Source: CAD feature listing. Evaluate the final solid. Frame: model axes, mm. A direction names the side the tool comes from. Give positions to 0.01 mm unless a question says otherwise; leave off trailing zeros. Write each loop counter-clockwise with the first axis right and the second up, starting at its lowest first coordinate (ties: lowest second). Pieces come first, ordered by that corner, then holes. Notation, with made-up numbers: (38.25, 26.5) -> (78.25, 26.5) arc R33 ccw to (78.25, 63.5) -> close; hole circle Ø10 at (70.5, 32). An arc over 180 degrees is marked (long way). Write item = value, one per line.
from build123d import *

# Parameters (mm, degrees)
SKETCH_W        = 18.5
SKETCH_H        = 18.5
PAD_DEPTH       = 5.5
SKETCH001_W     = 15.5
SKETCH001_H     = 15.5
POCKET_DEPTH    = 4
SKETCH002_R     = 2.7059
PAD001_DEPTH    = 4
POCKET001_DEPTH = 4
FILLET001_R     = 1.5
FILLET_R        = 2
PAD002_DEPTH    = 1.35295
FILLET002_R     = 1


with BuildPart() as part:
    # Sketch → Pad (new body)
    with BuildSketch(Plane.XY):
        Rectangle(SKETCH_W, SKETCH_H)
    extrude(amount=PAD_DEPTH)

    # Sketch001 → Pocket (cut)
    with BuildSketch(Plane(origin=(0, 0, 0), x_dir=(1, 0, 0), z_dir=(0, 0, -1))):
        Rectangle(SKETCH001_W, SKETCH001_H)
    extrude(amount=-POCKET_DEPTH, mode=Mode.SUBTRACT)

    # Sketch002 (on Face11 of Pocket) → Pad001 (join)
    with BuildSketch(Plane(origin=(0, 0, 4), x_dir=(1, 0, 0), z_dir=(0, 0, -1))):
        Circle(SKETCH002_R)
    extrude(amount=PAD001_DEPTH)

    # Sketch003 (on Face13 of Pad001) → Pocket001 (cut)
    with BuildSketch(Plane(origin=(0, 0, 0), x_dir=(1, 0, 0), z_dir=(0, 0, -1))):
        Polygon((-0.6219, 2.0443), (0.6219, 2.0443), (0.6219, 0.6219), (2.0443, 0.6219), (2.0443, -0.6219), (0.6219, -0.6219), (0.6219, -2.0443), (-0.6219, -2.0443), (-0.6219, -0.6219), (-2.0443, -0.6219), (-2.0443, 0.6219), (-0.6219, 0.6219), align=None)
    extrude(amount=-POCKET001_DEPTH, mode=Mode.SUBTRACT)

    # Fillet001
    fillet001_edges = [part.edges().sort_by_distance(p)[0] for p in [
        (-7.75, -7.75, 2),
        (7.75, -7.75, 2),
        (7.75, 7.75, 2),
        (-7.75, 7.75, 2),
    ]]
    fillet(fillet001_edges, radius=FILLET001_R)

    # Fillet
    fillet_edges = [part.edges().sort_by_distance(p)[0] for p in [
        (9.25, -9.25, 2.75),
        (-9.25, -9.25, 2.75),
        (-9.25, 9.25, 2.75),
        (9.25, 9.25, 2.75),
    ]]
    fillet(fillet_edges, radius=FILLET_R)

    # Sketch004 (on Face19 of Fillet) → Pad002 (join)
    with BuildSketch(Plane(origin=(0, 0, 4), x_dir=(1, 0, 0), z_dir=(0, 0, -1))):
        Polygon((-0.676475, 7.75), (0.676475, 7.75), (0.676475, 0.676475), (7.75, 0.676475), (7.75, -0.676475), (0.676475, -0.676475), (0.676475, -7.75), (-0.676475, -7.75), (-0.676475, -0.676475), (-7.75, -0.676475), (-7.75, 0.676475), (-0.676475, 0.676475), align=None)
    extrude(amount=PAD002_DEPTH)

    # Fillet002
    fillet002_edges = [part.edges().sort_by_distance(p)[0] for p in [
        (0, 9.25, 5.5),
        (-8.664214, 8.664214, 5.5),
        (8.664214, 8.664214, 5.5),
        (-9.25, 0, 5.5),
        (9.25, 0, 5.5),
        (-8.664214, -8.664214, 5.5),
        (8.664214, -8.664214, 5.5),
        (0, -9.25, 5.5),
    ]]
    fillet(fillet002_edges, radius=FILLET002_R)


solid = part.part
1) Draft query along X for faces 1 (the cylindrical face through (-0.101, -8.965, 5.199)), 2 (the cylindrical face through (-8.68, -8.65, 2.28)), 3 (the flat face through (2.044, 0, 1)). Return one class per face: pulls with the +X half, pulls with the -X half, needs draft (parallel to the pull), parting line crosses it, or undercut.
Computed:
face_1 = needs draft
face_2 = pulls with the -X half
face_3 = undercut
2) Contact query for flat-ended pins moving along their axis: pin 1 (0.7 mm diameter, centred on x = 0, y = 5, fed in from -Z); pin 2 (3.5 mm diameter, centred on x = 4.5, y = 5, fed in from -Z). Output: stop coordinate, or through.
Computed:
pin_1 = 2.65
pin_2 = 4
3) Cut plane A-A (z = 3.5). State how many separate pieces and enclosed holes the cut face has, then the cut area to 3 significant figures.
Computed:
separate_pieces = 1
enclosed_holes = 4
area = 151 mm²
4) Material intervals for L1, parallel to Y at x = -4.5, z = 3, sorted ascending.
Computed:
L1 = -9.25 to -7.75, -0.68 to 0.68, 7.75 to 9.25
5) Cut plane C-C (y = 0). Return the cut outline in (x, z).
Computed:
outline = (-9.25, 0) -> (-7.75, 0) -> (-7.75, 2.65) -> (-2.71, 2.65) -> (-2.71, 0) -> (-2.04, 0) -> (-2.04, 2.65) -> (2.04, 2.65) -> (2.04, 0) -> (2.71, 0) -> (2.71, 2.65) -> (7.75, 2.65) -> (7.75, 0) -> (9.25, 0) -> (9.25, 4.5) arc R1 ccw to (8.25, 5.5) -> (-8.25, 5.5) arc R1 ccw to (-9.25, 4.5) -> close
6) Access query for faces 4 (the flat face through (0, -7.75, 2)), 5 (the cylindrical face through (0.101, 8.965, 5.199)). Directions: +Z, -Z, +X, -X, +Y, -Y. A direction counts if a zero-diameter tool reaches every point of the face in a straight line with its end or side. Return the directions, or none.
Computed:
face_4 = -Z
face_5 = +Z, +X, -X, +Y
